```python
from build123d import *

# Parameters (mm, degrees)
SKETCH_1_W          = 80
SKETCH_1_H          = 60
EXTRUDE_1_DEPTH     = 40
CUT_EXTRUDE_1_DEPTH = 65.031242374
CUT_EXTRUDE_2_DEPTH = 65.031242374
SKETCH_4_W          = 10
SKETCH_4_H          = 60
CUT_EXTRUDE_3_DEPTH = 5
SKETCH_5_R          = 4
CUT_EXTRUDE_4_DEPTH = 12


with BuildPart() as part:
    # 草图1 → 凸台-拉伸1 (new body)
    with BuildSketch(Plane(origin=(0, 0, 0), x_dir=(1, 0, 0), z_dir=(0, 1, 0))):
        Rectangle(SKETCH_1_W, SKETCH_1_H)
    extrude(amount=EXTRUDE_1_DEPTH)

    # 草图2 → 切除-拉伸1 (cut, through all)
    with BuildSketch(Plane.XY):
        Polygon((-12, 0), (12, 0), (20.6603, 15), (-20.6603, 15), align=None)
    extrude(amount=CUT_EXTRUDE_1_DEPTH, mode=Mode.SUBTRACT)

    # 草图3 → 切除-拉伸2 (cut, through all)
    with BuildSketch(Plane.XY):
        Polygon((-12, 0), (12, 0), (20.6603, 15), (-20.6603, 15), align=None)
    extrude(amount=-CUT_EXTRUDE_2_DEPTH, mode=Mode.SUBTRACT)

    # 草图4 → 切除-拉伸3 (cut)
    with BuildSketch(Plane(origin=(0, 40, 0), x_dir=(1, 0, 0), z_dir=(0, 1, 0))):
        Rectangle(SKETCH_4_W, SKETCH_4_H)
    extrude(amount=-CUT_EXTRUDE_3_DEPTH, mode=Mode.SUBTRACT)

    # 草图5 → 切除-拉伸4 (cut)
    with BuildSketch(Plane(origin=(0, 40, 0), x_dir=(1, 0, 0), z_dir=(0, 1, 0))):
        with Locations(Location((-20, 0, 0), (0, 0, 270))):
            Circle(SKETCH_5_R)
        with Locations(Location((20, 0, 0), (0, 0, 270))):
            Circle(SKETCH_5_R)
    extrude(amount=-CUT_EXTRUDE_4_DEPTH, mode=Mode.SUBTRACT)


solid = part.part
```
Verification items for the finished model (mm, model axes). A direction names the side the tool comes from. Coordinates: 2 decimals unless noted, no trailing zeros. Write each loop counter-clockwise with the first axis right and the second up, starting at its lowest first coordinate (ties: lowest second). Pieces come first, ordered by that corner, then holes. Notation, with made-up numbers: M 32,76.5 L 75,76.5 A32 ccw 75,110.5 Z; hole C 26.25,3 d9. An arc over 180 degrees is marked long. Answer as a JSON object with one key per item and string values. Group by question number.
(1) Cross-section at D-D, the plane x = -6. Record the cut outline in (y, z), and give its area (3 significant figures).
(2) Cross-section at B-B, the plane z = 23. Record the cut outline in (x, y), and give its area (3 significant figures).
(3) Release check for a two-part mould opening along X. For faces 6 (the face through (40, 20, 0)), 7 (the face through (-20, 28, 0)), 8 (the face through (-27, 40, 0)) record: +X half, -X half, draft (parallel to the pull), parting line (faces both ways), or undercut.
(4) Cross-section at A-A, the plane y = 29.5. Record the cut outline in (x, z).
(5) Tool access check on faces 1 (the face through (23.966, 34.084, -0.521)), 2 (the face through (-40, 20, 0)), 3 (the face through (26, 40, 0)), 4 (the face through (16.27, 7.395, -0.42)), 5 (the face through (5, 38, 0)). Record the directions out of +Z, -Z, +X, -X, +Y, -Y that give a thin tool (end or side, any length) a straight path to the whole face; none if there is none.
(6) Gauge pin test, flat ends, axial feed: pin 1 (4 mm diameter, centred on x = -20, z = -0.5, fed in from +Y); pin 2 (8 mm diameter, centred on x = 0, z = 3, fed in from +Y). Record the tip position at first contact, or that the pin passes through.
(7) Cross-section at C-C, the plane y = 4.5. Record the cut outline in (x, z), and give its area (3 significant figures).
(8) Material ranges on line 1 (X direction, y = 37.75, z = 0); line 2 (X direction, y = 33.75, z = 0); line 3 (Y direction, x = -10, z = -20), recorded low to high.
Reply:
{
 "1": {"outline": "M 15,-30 L 40,-30 L 40,30 L 15,30 Z", "area": "1,500 mm²"},
 "2": {"outline": "M -40,0 L -12,0 L -20.66,15 L 20.66,15 L 12,0 L 40,0 L 40,40 L 5,40 L 5,35 L -5,35 L -5,40 L -40,40 Z", "area": "2,660 mm²"},
 "3": {"face 6": "+X half", "face 7": "undercut", "face 8": "draft"},
 "4": {"outline": "M -40,-30 L 40,-30 L 40,30 L -40,30 Z; hole C -20,0 d8; hole C 20,0 d8"},
 "5": {"face 1": "+Y", "face 2": "+Z, -Z, -X, +Y, -Y", "face 3": "+Z, -Z, +X, -X, +Y", "face 4": "+Z, -Z", "face 5": "+Z, -Z, +Y"},
 "6": {"pin 1": "y = 28", "pin 2": "y = 35"},
 "7": {"outline": "M -40,-30 L -14.6,-30 L -14.6,30 L -40,30 Z; M 14.6,-30 L 40,-30 L 40,30 L 14.6,30 Z", "area": "3,050 mm²"},
 "8": {"line 1": "-40 to -24, -16 to -5, 5 to 16, 24 to 40", "line 2": "-40 to -24, -16 to 16, 24 to 40", "line 3": "15 to 40"}
}
